Input: part model. Units: mm. Frame: model coordinates. Round coordinates to 2 decimals unless told otherwise and drop trailing zeros. Loops run counter-clockwise (first coordinate to the right, second up) from the corner with the lowest first, then second, coordinate; pieces in that order, holes last.
1) Draft query along Z for faces 1 (the face through (-56.19, -1.97, -91.66)), 2 (the face through (-78.334, -1.972, -107.893)), 3 (the face through (75.96, -1.97, -93.93)). Return one class per face: pulls with the +Z half, pulls with the -Z half, needs draft (parallel to the pull), parting line crosses it, or undercut.
2) Section A-A, the plane x = 57. Return loops of the section in (y, z).
3) Section C-C, the plane z = -79. Return loops of the section in (x, y).
4) Section B-B, the plane y = -2.8. Return loops of the section in (x, z), and give its area (3 significant figures).
5) Section D-D, the plane z = -97.5. Return loops of the section in (x, y), and give its area (3 significant figures).
6) Ray query, line 1 along X through (y, z) = (-0.7, -103.5); line 2 along X through (y, z) = (-2.25, -105.5); line 3 along Z through (x, y) = (-9.5, -1.3). Return the intervals inside material, ascending.
from build123d import *

# Parameters (mm, degrees)
F0_R     = 3
F1_DEPTH = 4


with BuildPart() as f1:
    # F0 (on Front) → F1 (new body)
    with BuildSketch(Plane.XZ):
        with BuildLine():
            ThreePointArc((48.885314, -75.566038), (0, -90), (-48.885314, -75.566038))
            ThreePointArc((-48.885314, -75.566038), (-62.959815, -73.932985), (-72.812289, -84.115676))
            Line((-72.812289, -84.115676), (-79.017923, -103.473649))
            ThreePointArc((-79.017923, -103.473649), (-78.295886, -107.946883), (-74.256595, -110))
            Line((-74.256595, -110), (32.693748, -110))
            Line((32.693748, -110), (61.95706, -110))
            Line((61.95706, -110), (74.256595, -110))
            ThreePointArc((74.256595, -110), (78.295886, -107.946883), (79.017923, -103.473649))
            Line((79.017923, -103.473649), (72.812289, -84.115676))
            ThreePointArc((72.812289, -84.115676), (62.959815, -73.932985), (48.885314, -75.566038))
        make_face()
        with Locations((-57.576037, -89)):
            Circle(F0_R, mode=Mode.SUBTRACT)
        with Locations((57.576037, -89)):
            Circle(F0_R, mode=Mode.SUBTRACT)
    extrude(amount=F1_DEPTH)


solid = f1.part
Final values:
1. face 1: undercut
1. face 2: parting line crosses it
1. face 3: pulls with the +Z half
2. outline: (-4, -110) - (0, -110) - (0, -91.94) - (-4, -91.94) - close; (-4, -86.06) - (0, -86.06) - (0, -73.01) - (-4, -73.01) - close
3. outline: (-70.07, -4) - (-43.12, -4) - (-43.12, 0) - (-70.07, 0) - close; (43.12, -4) - (70.07, -4) - (70.07, 0) - (43.12, 0) - close
4. outline: (-79.02, -103.47) arc R5 ccw to (-74.26, -110) - (74.26, -110) arc R5 ccw to (79.02, -103.47) - (72.81, -84.12) arc R16 ccw to (48.89, -75.57) arc R90 cw to (-48.89, -75.57) arc R16 ccw to (-72.81, -84.12) - close; hole circle Ø6 at (-57.58, -89); hole circle Ø6 at (57.58, -89)
4. area: 4,210 mm2
5. outline: (-77.1, -4) - (77.1, -4) - (77.1, 0) - (-77.1, 0) - close
5. area: 617 mm2
6. line 1: x = -79.03 to 79.03
6. line 2: x = -79.23 to 79.23
6. line 3: z = -110 to -89.5
